Geometry: final body of the model. Coordinates: model frame, mm. A direction names the side the tool comes from. Coordinates: 2 decimals unless noted, no trailing zeros. Order: outer loops, then holes, each group sorted by start corner. A loop starts at its lowest first (then second) coordinate and runs counter-clockwise, first axis right, second up. Notation, with made-up numbers: M 34,-37.75 L 41,-37.75 A23 cw 41,-4.75 Z; hole C 15,23 d10. An arc over 180 degrees is marked long. Use CSV: the item, a comma, the result in double quotes. Start each with the question number.
Q1. Section query B-B, the plane x = 100. Output: boundary loops of the cut face in (y, z) (3 decimals).
Q2. Mould query, pull axis Z, two halves, no side actions, for faces 1 (the face through (148.94, -8.15, 0.33)), 2 (the face through (-19.05, 0, 0)), 3 (the face through (122, 6.985, 0)). Classes: +Z half, -Z half, draft (parallel to the pull), parting line (faces both ways), or undercut.
Q3. Ray query, probe 1 along X at (y, z) = (3.75, -4.25) (3 decimals); probe 2 along Z at (x, y) = (97.5, 8.5); probe 3 along Z at (x, y) = (37.5, 4). Return the intervals inside material, ascending.
Q4. Section query C-C, the plane x = 53. Output: boundary loops of the cut face in (y, z) (3 decimals).
Q5. First-contact query: P1, Ø1.1, axis at x = 11, z = 8.5, coming from the -Y side; P2, Ø1.8, axis at x = 10, z = 8.5, coming from the +Y side; P3, Ø1.5, axis at x = 149, z = -4.5, coming from the -Y side; P4, Ø6, axis at x = 91, z = -1.5, coming from the -Y side (3 decimals). Flat tips, straight axial feed; report the tip coordinate or a pass-through.
Q6. Access query for faces 4 (the face through (-9, 3.175, 0)), 5 (the face through (15, 0, 6.985)), 6 (the face through (168.275, 0, 0)), 7 (the face through (158.046, -1.431, 4.543)), 8 (the face through (-8.58, -4.76, 0.15)). Directions: +Z, -Z, +X, -X, +Y, -Y. A direction counts if a zero-diameter tool reaches every point of the face in a straight line with its end or side. Return the directions, or none.
from build123d import *

# Parameters (mm, degrees)
BOSS_EXTRUDE1_DEPTH = 19.05
CUT_EXTRUDE1_START  = 6.985
CUT_EXTRUDE1_DEPTH  = 19.05
CUT_EXTRUDE2_START  = 6.985
CUT_EXTRUDE2_DEPTH  = 19.05


with BuildPart() as part:
    # Sketch1 → Revolve1 (revolve)
    with BuildSketch(Plane.XY, mode=Mode.PRIVATE) as revolve1_sk:
        Polygon((0, 0), (0, 9.525), (149.225, 9.525), (149.225, 4.7625), (168.275, 4.7625), (168.275, 0), align=None)
    revolve(revolve1_sk.sketch.rotate(Axis((0, 0, 0), (1, 0, 0)), 90), axis=Axis((0, 0, 0), (1, 0, 0)))

    # Sketch2 → Boss-Extrude1 (add)
    with BuildSketch(Plane.ZY):
        with BuildLine():
            Line((-3.549757914, 3.175), (3.549757914, 3.175))
            ThreePointArc((3.549757914, 3.175), (0, -4.7625), (-3.549757914, 3.175))
        make_face()
    extrude(amount=BOSS_EXTRUDE1_DEPTH)

    # Chamfer1: read off the stored shape, not the designer's step
    # Chamfer1 outline → Chamfer1 (revolve, cut)
    with BuildSketch(Plane.YX):
        Polygon((4.7625, 168.275), (3.1115, 168.275), (4.7625, 166.624), align=None)
        Polygon((9.525, 149.225), (7.874, 149.225), (9.525, 147.574), align=None)
        Polygon((9.525, 0), (9.525, 1.651), (7.874, 0), align=None)
        Polygon((4.7625, -19.05), (4.7625, -17.399), (3.1115, -19.05), align=None)
    revolve(axis=Axis((0, 0, 0), (1, 0, 0)), mode=Mode.SUBTRACT)

    # Sketch4 → Cut-Extrude1 (cut)
    with BuildSketch(Plane.XY.offset(CUT_EXTRUDE1_START)):
        with BuildLine():
            Line((0, 2.38125), (0, -2.38125))
            Line((0, -2.38125), (28.575, -2.38125))
            ThreePointArc((28.575, -2.38125), (30.95625, 0), (28.575, 2.38125))
            Line((28.575, 2.38125), (0, 2.38125))
        make_face()
    extrude(amount=CUT_EXTRUDE1_DEPTH, mode=Mode.SUBTRACT)

    # Sketch5 → Cut-Extrude2 (cut)
    with BuildSketch(Plane(origin=(0, 0, 0), x_dir=(1, 0, 0), z_dir=(0, 1, 0)).offset(CUT_EXTRUDE2_START)):
        with BuildLine():
            Line((149.225, 2.38125), (149.225, -2.38125))
            Line((149.225, -2.38125), (96.8248, -2.38125))
            ThreePointArc((96.8248, -2.38125), (94.44355, 0), (96.8248, 2.38125))
            Line((96.8248, 2.38125), (149.225, 2.38125))
        make_face()
    extrude(amount=CUT_EXTRUDE2_DEPTH, mode=Mode.SUBTRACT)


solid = part.part
Responses:
1,outline,"M 6.985,-2.381 L 6.985,2.381 L 9.223,2.381 A9.525 ccw long 9.223,-2.381 Z"
2,face 1,"parting line"
2,face 2,"draft"
2,face 3,"undercut"
3,probe 1,"x = 0 to 149.225"
3,probe 2,"z = -4.3 to -2.38, 2.38 to 4.3"
3,probe 3,"z = -8.64 to 8.64"
4,outline,"C 0,0 d19.05"
5,P1,"stops at y = -5.25"
5,P2,"stops at y = 5.74"
5,P3,"stops at y = -7.72"
5,P4,"stops at y = -9.525"
6,face 4,"+Z, -Z, -X, +Y"
6,face 5,"+Z, -X"
6,face 6,"+Z, -Z, +X, +Y, -Y"
6,face 7,"+X"
6,face 8,"-X"
